Part model, mm, in its own coordinate system. A direction names the side the tool comes from. Give positions to 0.01 mm unless a question says otherwise; leave off trailing zeros. Write item = value, one per line. Start each with the question number.
(1) Flat gauge pins, fed straight in: pin 1 (2 mm diameter, centred on x = 69.5, z = 4, fed in from +Y); pin 2 (25 mm diameter, centred on y = -102.5, z = 12, fed in from -X); pin 3 (1 mm diameter, centred on x = 44, z = 30.5, fed in from -Y). Where does each tip first touch, or does it go through?
(2) Saw through at A-A, the plane y = -80. State how many separate pieces and enclosed holes the cut face has, then the cut area to 3 significant figures.
(3) Two-plate mould, pull along Z, no slides. Class faces 1 (the flat face through (-107.15, 0, 0)), 2 (the flat face through (0, 117, 47.5)), 3 (the flat face through (-0.39, 118.78, 45.77)): pulls with the +Z half, pulls with the -Z half, needs draft (parallel to the pull), parting line crosses it, or undercut.
(4) Which spindle directions (+Z, -Z, +X, -X, +Y, -Y) get a long thin tool onto all of the face, cutting with end or side? Do faces 4 (the flat face through (109, 183, -46)), 5 (the flat face through (110.65, 0, 0)). Say none if no direction does.
(5) Probe line 1 along Y through (x, z) = (3, -21); line 2 along X through (y, z) = (62.5, -47.75); line 3 along X through (y, z) = (-152, 42.5). List the from-to ranges inside material, lowest first. Write a range as from..to.
from build123d import *

# Parameters (mm, degrees)
SKETCH2_W               = 226.3
SKETCH2_H               = 100
BOSS_EXTRUDE1_DEPTH     = 183
SKETCH4_OUTSIDE_W       = 316.656
SKETCH4_OUTSIDE_H       = 190.356
SKETCH4_OUTSIDE_W_2     = 8.5
SKETCH4_OUTSIDE_H_2     = 8.5
CUT_EXTRUDE1_DEPTH      = 6
SKETCH5_W               = 209.3
SKETCH5_H               = 114
CUT_EXTRUDE2_DEPTH      = 238.259188442
SKETCH6_W               = 83
SKETCH6_H               = 114
CUT_EXTRUDE3_DEPTH      = 296.29762952
EXTRUDE_THIN1_START     = -2.5
EXTRUDE_THIN1_DEPTH     = 3.5
EXTRUDE_THIN2_START     = -2.5
EXTRUDE_THIN2_DEPTH     = 3.5
CIRPATTERN1_COUNT       = 2
DELETEFACE2_START       = 107.15
DELETEFACE2_DEPTH       = 3.5
CUT_EXTRUDE4_DEPTH      = 221.888937025
CUT_EXTRUDE4_DEPTH_BACK = 221.888937025
SKETCH9_R               = 1.25


# Read off the part's stored shape, not the designer's step: DeleteFace2
with BuildPart() as part:
    # Sketch2 → Boss-Extrude1 (new, symmetric)
    with BuildSketch(Plane(origin=(0, 0, 0), x_dir=(1, 0, 0), z_dir=(0, 1, 0))):
        Rectangle(SKETCH2_W, SKETCH2_H)
    extrude(amount=BOSS_EXTRUDE1_DEPTH, both=True)

    # Sketch4 outside → Cut-Extrude1 (cut)
    with BuildSketch(Plane.XZ.offset(183)):
        Rectangle(SKETCH4_OUTSIDE_W, SKETCH4_OUTSIDE_H)
        with Locations((-108.9, 45.75)):
            Rectangle(SKETCH4_OUTSIDE_W_2, SKETCH4_OUTSIDE_H_2, mode=Mode.SUBTRACT)
        with Locations((-108.9, -45.75)):
            Rectangle(SKETCH4_OUTSIDE_W_2, SKETCH4_OUTSIDE_H_2, mode=Mode.SUBTRACT)
        with Locations((108.9, -45.75)):
            Rectangle(SKETCH4_OUTSIDE_W_2, SKETCH4_OUTSIDE_H_2, mode=Mode.SUBTRACT)
        with Locations((108.9, 45.75)):
            Rectangle(SKETCH4_OUTSIDE_W_2, SKETCH4_OUTSIDE_H_2, mode=Mode.SUBTRACT)
    cut_extrude1 = extrude(amount=-CUT_EXTRUDE1_DEPTH, mode=Mode.SUBTRACT)

    # Mirror1: Cut-Extrude1 across plane
    add(cut_extrude1.mirror(Plane.ZX), mode=Mode.SUBTRACT)

    # Sketch5 → Cut-Extrude2 (cut, through all)
    with BuildSketch(Plane.XY.offset(50)):
        with Locations((0, 117)):
            Rectangle(SKETCH5_W, SKETCH5_H)
        with Locations((0, -117)):
            Rectangle(SKETCH5_W, SKETCH5_H)
        Rectangle(SKETCH5_W, SKETCH5_H)
    extrude(amount=-CUT_EXTRUDE2_DEPTH, mode=Mode.SUBTRACT)

    # Sketch6 → Cut-Extrude3 (cut, through all)
    with BuildSketch(Plane(origin=(113.15, 0, 0), x_dir=(0, 0, -1), z_dir=(1, 0, 0))):
        with Locations((0, 117)):
            Rectangle(SKETCH6_W, SKETCH6_H)
        with Locations((0, -117)):
            Rectangle(SKETCH6_W, SKETCH6_H)
        Rectangle(SKETCH6_W, SKETCH6_H)
    extrude(amount=-CUT_EXTRUDE3_DEPTH, mode=Mode.SUBTRACT)

    # Sketch7 → Extrude-Thin1 (add)
    with BuildSketch(Plane.XY.offset(50).offset(EXTRUDE_THIN1_START)):
        Polygon((-103.812934943, -175.536822075), (105.487065057, -61.536822075), (103.812934943, -58.463177925), (-105.487065057, -172.463177925), align=None)
        Polygon((-103.812934943, -58.536822075), (105.487065057, 55.463177925), (103.812934943, 58.536822075), (-105.487065057, -55.463177925), align=None)
        Polygon((-103.812934943, 58.463177925), (105.487065057, 172.463177925), (103.812934943, 175.536822075), (-105.487065057, 61.536822075), align=None)
    extrude_thin1 = extrude(amount=-EXTRUDE_THIN1_DEPTH)

    # Sketch8 → Extrude-Thin2 (add)
    with BuildSketch(Plane(origin=(113.15, 0, 0), x_dir=(0, 0, -1), z_dir=(1, 0, 0)).offset(EXTRUDE_THIN2_START)):
        Polygon((-40.085248698, -175.030038229), (42.914751302, -61.030038229), (40.085248698, -58.969961771), (-42.914751302, -172.969961771), align=None)
        Polygon((-40.085248698, -58.030038229), (42.914751302, 55.969961771), (40.085248698, 58.030038229), (-42.914751302, -55.969961771), align=None)
        Polygon((-40.085248698, 58.969961771), (42.914751302, 172.969961771), (40.085248698, 175.030038229), (-42.914751302, 61.030038229), align=None)
    extrude_thin2 = extrude(amount=-EXTRUDE_THIN2_DEPTH)

    # CirPattern1: Extrude-Thin1, Extrude-Thin2 ×2 about axis
    cirpattern1_axis = Axis((0, 0, 0), (0, 1, 0))
    add([extrude_thin1.rotate(cirpattern1_axis, i * 360 / CIRPATTERN1_COUNT) for i in range(1, CIRPATTERN1_COUNT)])
    add([extrude_thin2.rotate(cirpattern1_axis, i * 360 / CIRPATTERN1_COUNT) for i in range(1, CIRPATTERN1_COUNT)])

    # DeleteFace2 outline → DeleteFace2 (cut)
    with BuildSketch(Plane.YZ.offset(DELETEFACE2_START)):
        Polygon((60, 41.5), (60, 39.335308584), (171.02680938, -41.5), (174, -41.5), (174, -39.335308584), (62.97319062, 41.5), align=None)
    extrude(amount=DELETEFACE2_DEPTH, mode=Mode.SUBTRACT)

    # Sketch9 → Cut-Extrude4 (cut, two sides: drawn at the far end of the back side and taken through both)
    with BuildSketch(Plane.XY.offset(-CUT_EXTRUDE4_DEPTH_BACK)):
        with Locations((108.9, 62.5)):
            Circle(SKETCH9_R)
    extrude(amount=CUT_EXTRUDE4_DEPTH + CUT_EXTRUDE4_DEPTH_BACK, mode=Mode.SUBTRACT)


solid = part.part
Results list:
q1.pin_1 = 177
q1.pin_2 = -110.65
q1.pin_3 = -177
q2.separate_pieces = 8
q2.enclosed_holes = 0
q2.area = 371 mm^2
q3.face_1 = undercut
q3.face_2 = pulls with the +Z half
q3.face_3 = needs draft
q4.face_4 = +Z, -Z, +X, -X, +Y
q4.face_5 = +X
q5.line_1 = -177..-174, -60..-57, 57..60, 174..177
q5.line_2 = -113.15..-104.65, 104.65..107.65, 110.15..113.15
q5.line_3 = -113.15..-104.65, 104.65..113.15
